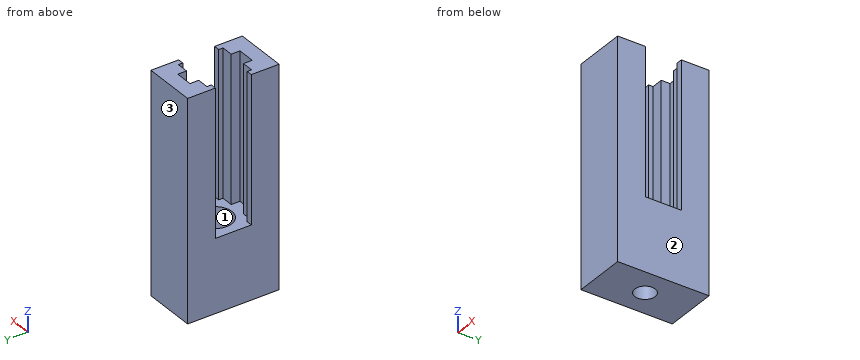
from build123d import *

# Parameters (mm, degrees)
BOSS_EXTRUDE1_DEPTH = 50
SKETCH3_W           = 18
SKETCH3_H           = 31.3
BOSS_EXTRUDE2_DEPTH = 25
SKETCH4_R           = 5.75
CUT_EXTRUDE1_DEPTH  = 16
SKETCH5_R           = 3.5
CUT_EXTRUDE2_DEPTH  = 10


with BuildPart() as part:
    # Sketch2 → Boss-Extrude1 (new body)
    with BuildSketch(Plane.XY):
        Polygon((-3, -10.65), (3, -10.65), (3, -7.65), (7, -7.65), (7, -6.15), (9, -6.15), (9, -7.65), (9, -15.65), (-9, -15.65), (-9, -7.65), (-9, -6.15), (-7, -6.15), (-7, -7.65), (-3, -7.65), align=None)
    extrude(amount=BOSS_EXTRUDE1_DEPTH)


with BuildPart() as body_2:
    # Mirror2: mirrored copy
    add(part.part.mirror(Plane.ZX))


with BuildPart() as part_1:
    add(part.part)

    add(body_2.part)  # Boss-Extrude2 merges body 2
    # Sketch3 → Boss-Extrude2 (add)
    with BuildSketch(Plane(origin=(0, 0, 0), x_dir=(-1, 0, 0), z_dir=(0, 0, -1))):
        Rectangle(SKETCH3_W, SKETCH3_H)
    extrude(amount=BOSS_EXTRUDE2_DEPTH)

    # Sketch4 → Cut-Extrude1 (cut)
    with BuildSketch(Plane.XY):
        Circle(SKETCH4_R)
    extrude(amount=-CUT_EXTRUDE1_DEPTH, mode=Mode.SUBTRACT)

    # Sketch5 → Cut-Extrude2 (cut, through all)
    with BuildSketch(Plane.XY.offset(-16)):
        Circle(SKETCH5_R)
    extrude(amount=-CUT_EXTRUDE2_DEPTH, mode=Mode.SUBTRACT)


solid = part_1.part
Could you check a few things on this model? Use its own coordinates, in mm. Face numbers are marked on the shaded views. Coordinates: 2 decimals unless noted, no trailing zeros. Order: outer loops, then holes, each group sorted by start corner. A loop starts at its lowest first (then second) coordinate and runs counter-clockwise, first axis right, second up. Notation, with made-up numbers: (-12, 30.5) - (14, 30.5) arc R21 cw to (14, 35.5) - close; hole circle Ø6 at (-5, 24.5). An arc over 180 degrees is marked (long way). Answer in a Markdown table with one row per item. Add a question column.
(1) Will these pins go through, and if not, where does the flat tip stop? pin 1 (9 mm diameter, centred on x = 0, y = 0, fed in from +Z); pin 2 (5.5 mm diameter, centred on x = -2, y = -5, fed in from +Z).
(2) If we mould it in two halves opening along Y, with no side actions, what happens to the marked faces 1, 2 and 3? For each: released by +Y, released by -Y, zero draft, split by the parting line, or undercut.
(3) If we section it at C-C, the plane z = 21: Please give me the cut outline in (x, y), then the cut area to 3 significant figures.
(4) If we section it at A-A, the plane y = 0: Please give me the cut outline in (x, z).
(5) If we section it at D-D, the plane z = -13: Please give me the cut outline in (x, y), then the cut area to 3 significant figures.
(6) I need wall thicknesses on L1, parallel to Y at x = 0, z = -20.5; L2, parallel to Y at x = 0, z = -4.5; L3, parallel to Z at x = -6.5, y = 2. Which ranges of each line are inside material? Lowest first, please.
(7) If we section it at B-B, the plane x = 0: Please give me the cut outline in (y, z).
Results are:
| question | item | result |
|---|---|---|
| 1 | pin 1 | stops at z = -16 |
| 1 | pin 2 | stops at z = 0 |
| 2 | face 1 | undercut |
| 2 | face 2 | zero draft |
| 2 | face 3 | released by +Y |
| 3 | outline | (-9, -15.65) - (9, -15.65) - (9, -6.15) - (7, -6.15) - (7, -7.65) - (3, -7.65) - (3, -10.65) - (-3, -10.65) - (-3, -7.65) - (-7, -7.65) - (-7, -6.15) - (-9, -6.15) - close; (-9, 6.15) - (-7, 6.15) - (-7, 7.65) - (-3, 7.65) - (-3, 10.65) - (3, 10.65) - (3, 7.65) - (7, 7.65) - (7, 6.15) - (9, 6.15) - (9, 15.65) - (-9, 15.65) - close |
| 3 | area | 264 mm2 |
| 4 | outline | (-9, -25) - (-3.5, -25) - (-3.5, -16) - (-5.75, -16) - (-5.75, 0) - (-9, 0) - close; (3.5, -25) - (9, -25) - (9, 0) - (5.75, 0) - (5.75, -16) - (3.5, -16) - close |
| 5 | outline | (-9, -15.65) - (9, -15.65) - (9, 15.65) - (-9, 15.65) - close; hole circle Ø11.5 at (0, 0) |
| 5 | area | 460 mm2 |
| 6 | L1 | y = -15.65 to -3.5, 3.5 to 15.65 |
| 6 | L2 | y = -15.65 to -5.75, 5.75 to 15.65 |
| 6 | L3 | z = -25 to 0 |
| 7 | outline | (-15.65, -25) - (-3.5, -25) - (-3.5, -16) - (-5.75, -16) - (-5.75, 0) - (-10.65, 0) - (-10.65, 50) - (-15.65, 50) - close; (3.5, -25) - (15.65, -25) - (15.65, 50) - (10.65, 50) - (10.65, 0) - (5.75, 0) - (5.75, -16) - (3.5, -16) - close |
